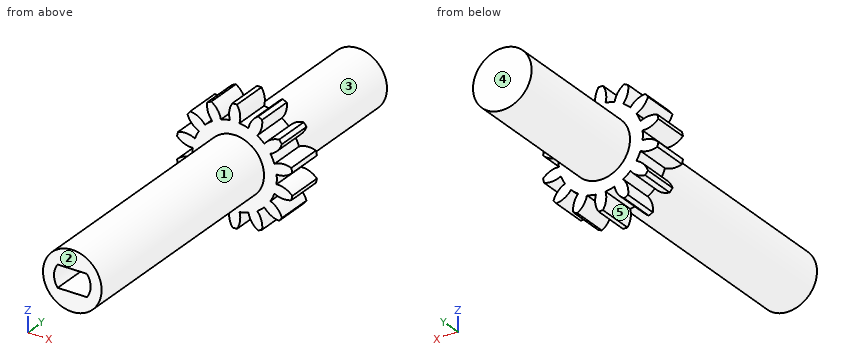
```python
from build123d import *

# Parameters (mm, degrees)
SKETCH1_R                = 0.4
BOSS_EXTRUDE1_DEPTH      = 5
BOSS_EXTRUDE2_DEPTH      = 33
BOSS_EXTRUDE2_DEPTH_BACK = 5
SKETCH2_R                = 4
BOSS_EXTRUDE3_START      = 20
SKETCH3_R                = 4
BOSS_EXTRUDE3_DEPTH      = 20
CUT_EXTRUDE1_DEPTH       = 33


with BuildPart() as part:
    # Sketch1 → Boss-Extrude1 (new body)
    with BuildSketch(Plane(origin=(0, 0, 0), x_dir=(1, 0, 0), z_dir=(0, 1, 0))):
        with BuildLine():
            ThreePointArc((3.744900382, -7.069350828), (3.64692573, -5.891768521), (3.071904032, -4.859465672))
            ThreePointArc((3.071904032, -4.859465672), (3.584442871, -4.494749193), (4.054065768, -4.076217824))
            ThreePointArc((4.054065768, -4.076217824), (4.932532263, -4.866531521), (6.058788713, -5.224086459))
            ThreePointArc((6.058788713, -5.224086459), (6.25465186, -4.987918415), (6.441315028, -4.744413632))
            ThreePointArc((6.441315028, -4.744413632), (5.842109102, -3.725958242), (4.876133034, -3.045378078))
            ThreePointArc((4.876133034, -3.045378078), (5.179670022, -2.494397616), (5.421191676, -1.913552144))
            ThreePointArc((5.421191676, -1.913552144), (6.555566902, -2.244447854), (7.725426174, -2.077929362))
            ThreePointArc((7.725426174, -2.077929362), (7.799423297, -1.780167472), (7.861948235, -1.47978713))
            ThreePointArc((7.861948235, -1.47978713), (6.880191117, -0.822176238), (5.714584087, -0.628116006))
            ThreePointArc((5.714584087, -0.628116006), (5.749, 0), (5.714584087, 0.628116006))
            ThreePointArc((5.714584087, 0.628116006), (6.880191117, 0.822176238), (7.861948235, 1.47978713))
            ThreePointArc((7.861948235, 1.47978713), (7.799423297, 1.780167472), (7.725426174, 2.077929362))
            ThreePointArc((7.725426174, 2.077929362), (6.555566902, 2.244447854), (5.421191676, 1.913552144))
            ThreePointArc((5.421191676, 1.913552144), (5.179670022, 2.494397616), (4.876133034, 3.045378078))
            ThreePointArc((4.876133034, 3.045378078), (5.842109102, 3.725958242), (6.441315028, 4.744413632))
            ThreePointArc((6.441315028, 4.744413632), (6.25465186, 4.987918415), (6.058788713, 5.224086459))
            ThreePointArc((6.058788713, 5.224086459), (4.932532263, 4.866531521), (4.054065768, 4.076217824))
            ThreePointArc((4.054065768, 4.076217824), (3.584442871, 4.494749193), (3.071904032, 4.859465672))
            ThreePointArc((3.071904032, 4.859465672), (3.64692573, 5.891768521), (3.744900382, 7.069350828))
            ThreePointArc((3.744900382, 7.069350828), (3.471069913, 7.207750943), (3.192133841, 7.335549164))
            ThreePointArc((3.192133841, 7.335549164), (2.332549116, 6.524738937), (1.883982415, 5.431538572))
            ThreePointArc((1.883982415, 5.431538572), (1.279272849, 5.604860567), (0.659246762, 5.711076493))
            ThreePointArc((0.659246762, 5.711076493), (0.72942399, 6.890641786), (0.306762287, 7.994116393))
            ThreePointArc((0.306762287, 7.994116393), (0, 8), (-0.306762287, 7.994116393))
            ThreePointArc((-0.306762287, 7.994116393), (-0.72942399, 6.890641786), (-0.659246762, 5.711076493))
            ThreePointArc((-0.659246762, 5.711076493), (-1.279272849, 5.604860567), (-1.883982415, 5.431538572))
            ThreePointArc((-1.883982415, 5.431538572), (-2.332549116, 6.524738937), (-3.192133841, 7.335549164))
            ThreePointArc((-3.192133841, 7.335549164), (-3.471069913, 7.207750943), (-3.744900382, 7.069350828))
            ThreePointArc((-3.744900382, 7.069350828), (-3.64692573, 5.891768521), (-3.071904032, 4.859465672))
            ThreePointArc((-3.071904032, 4.859465672), (-3.584442871, 4.494749193), (-4.054065768, 4.076217824))
            ThreePointArc((-4.054065768, 4.076217824), (-4.932532263, 4.866531521), (-6.058788713, 5.224086459))
            ThreePointArc((-6.058788713, 5.224086459), (-6.25465186, 4.987918415), (-6.441315028, 4.744413632))
            ThreePointArc((-6.441315028, 4.744413632), (-5.842109102, 3.725958242), (-4.876133034, 3.045378078))
            ThreePointArc((-4.876133034, 3.045378078), (-5.179670022, 2.494397616), (-5.421191676, 1.913552144))
            ThreePointArc((-5.421191676, 1.913552144), (-6.555566902, 2.244447854), (-7.725426174, 2.077929362))
            ThreePointArc((-7.725426174, 2.077929362), (-7.799423297, 1.780167472), (-7.861948235, 1.47978713))
            ThreePointArc((-7.861948235, 1.47978713), (-6.880191117, 0.822176238), (-5.714584087, 0.628116006))
            ThreePointArc((-5.714584087, 0.628116006), (-5.749, 0), (-5.714584087, -0.628116006))
            ThreePointArc((-5.714584087, -0.628116006), (-6.880191117, -0.822176238), (-7.861948235, -1.47978713))
            ThreePointArc((-7.861948235, -1.47978713), (-7.799423297, -1.780167472), (-7.725426174, -2.077929362))
            ThreePointArc((-7.725426174, -2.077929362), (-6.555566902, -2.244447854), (-5.421191676, -1.913552144))
            ThreePointArc((-5.421191676, -1.913552144), (-5.179670022, -2.494397616), (-4.876133034, -3.045378078))
            ThreePointArc((-4.876133034, -3.045378078), (-5.842109102, -3.725958242), (-6.441315028, -4.744413632))
            ThreePointArc((-6.441315028, -4.744413632), (-6.25465186, -4.987918415), (-6.058788713, -5.224086459))
            ThreePointArc((-6.058788713, -5.224086459), (-4.932532263, -4.866531521), (-4.054065768, -4.076217824))
            ThreePointArc((-4.054065768, -4.076217824), (-3.584442871, -4.494749193), (-3.071904032, -4.859465672))
            ThreePointArc((-3.071904032, -4.859465672), (-3.64692573, -5.891768521), (-3.744900382, -7.069350828))
            ThreePointArc((-3.744900382, -7.069350828), (-3.471069913, -7.207750943), (-3.192133841, -7.335549164))
            ThreePointArc((-3.192133841, -7.335549164), (-2.332549116, -6.524738937), (-1.883982415, -5.431538572))
            ThreePointArc((-1.883982415, -5.431538572), (-1.279272849, -5.604860567), (-0.659246762, -5.711076493))
            ThreePointArc((-0.659246762, -5.711076493), (-0.72942399, -6.890641786), (-0.306762287, -7.994116393))
            ThreePointArc((-0.306762287, -7.994116393), (0, -8), (0.306762287, -7.994116393))
            ThreePointArc((0.306762287, -7.994116393), (0.72942399, -6.890641786), (0.659246762, -5.711076493))
            ThreePointArc((0.659246762, -5.711076493), (1.279272849, -5.604860567), (1.883982415, -5.431538572))
            ThreePointArc((1.883982415, -5.431538572), (2.332549116, -6.524738937), (3.192133841, -7.335549164))
            ThreePointArc((3.192133841, -7.335549164), (3.471069913, -7.207750943), (3.744900382, -7.069350828))
        make_face()
        with Locations(Location((0, 0, 0), (0, 0, 90))):
            Circle(SKETCH1_R, mode=Mode.SUBTRACT)
    extrude(amount=-BOSS_EXTRUDE1_DEPTH)

    # Sketch2 → Boss-Extrude2 (add, two sides: drawn at the far end of the back side and taken through both)
    with BuildSketch(Plane.XZ.offset(5).offset(-BOSS_EXTRUDE2_DEPTH_BACK)):
        with Locations(Location((0, 0, 0), (0, 0, 270))):
            Circle(SKETCH2_R)
    extrude(amount=BOSS_EXTRUDE2_DEPTH + BOSS_EXTRUDE2_DEPTH_BACK)

    # Sketch3 → Boss-Extrude3 (add)
    with BuildSketch(Plane(origin=(0, 0, 0), x_dir=(1, 0, 0), z_dir=(0, 1, 0)).offset(BOSS_EXTRUDE3_START)):
        with Locations(Location((0, 0, 0), (0, 0, 90))):
            Circle(SKETCH3_R)
    extrude(amount=-BOSS_EXTRUDE3_DEPTH)

    # Sketch4 → Cut-Extrude1 (cut)
    with BuildSketch(Plane.XZ.offset(38)):
        with BuildLine():
            Line((-2, -1.5), (2, -1.5))
            ThreePointArc((2, -1.5), (2.5, 0), (2, 1.5))
            Line((2, 1.5), (-2, 1.5))
            ThreePointArc((-2, 1.5), (-2.5, 0), (-2, -1.5))
        make_face()
    extrude(amount=-CUT_EXTRUDE1_DEPTH, mode=Mode.SUBTRACT)


solid = part.part
```
The model under review builds one solid part; all positions refer to its coordinate system, in mm. Face numbers are marked on the shaded views. A direction names the side the tool comes from. Give positions to 0.01 mm unless a question says otherwise; leave off trailing zeros. Loops run counter-clockwise (first coordinate to the right, second up) from the corner with the lowest first, then second, coordinate; pieces in that order, holes last. Notation, with made-up numbers: (10.5, 32.25) - (24.5, 32.25) arc R18 cw to (24.5, 47.25) - close; hole circle Ø5 at (84.5, 21). An arc over 180 degrees is marked (long way). Answer as a JSON object with one key per item and string values.
Q1. Add section C-C on y = 14.5. State the section outline as (x, z) points.
Worked out:
{"outline": "circle Ø8 at (0, 0)"}
Q2. To check wall thickness, follow line 1 along X through (y, z) = (-2, 7); line 2 along X through (y, z) = (-3, 5.75); line 3 along Y through (x, z) = (-2, -4.25). State the ranges of each line that lie inside material, in increasing order.
Worked out:
{"line 1": "x = -3.75 to -2.74, -0.71 to 0.71, 2.74 to 3.75", "line 2": "x = -3.6 to -1.96, -0.67 to 0.67, 1.96 to 3.6", "line 3": "y = -5 to 0"}
Q3. Insertion check: pin 1 (8 mm diameter, centred on x = 5.5, y = -6.5, fed in from +Z); pin 2 (2 mm diameter, centred on y = -9, z = -1.5, fed in from -X); pin 3 (1 mm diameter, centred on y = -4.5, z = -5.5, fed in from +X) (3 decimals). Each pin has a flat end and moves straight along its axis. Give the tip position at first contact, or say it passes through.
Worked out:
{"pin 1": "stops at z = 7.34", "pin 2": "stops at x = -3.97", "pin 3": "stops at x = 6.245"}
Q4. Mouldability with a two-part tool opening along X and no side actions: class the marked faces 3, 4 and 5 as +X half, -X half, draft (parallel to the pull), parting line (faces both ways), or undercut.
Worked out:
{"face 3": "parting line", "face 4": "draft", "face 5": "undercut"}
Q5. Add section B-B on z = 0. State the section outline as (x, y) points, plus the area to 3 significant figures.
Worked out:
{"outline": "(-5.75, -5) - (-4, -5) - (-4, -38) - (-2.5, -38) - (-2.5, -5) - (2.5, -5) - (2.5, -38) - (4, -38) - (4, -5) - (5.75, -5) - (5.75, 0) - (4, 0) - (4, 20) - (-4, 20) - (-4, 0) - (-5.75, 0) - close", "area": "316 mm^2"}
Q6. For the marked faces 1 and 2, list the 3-axis set-ups (+Z, -Z, +X, -X, +Y, -Y) from which the entire face can be reached by the end or side of a thin tool; tool diameter is ignored.
Worked out:
{"face 1": "-Y", "face 2": "+Z, -Z, +X, -X, -Y"}
Q7. Add section A-A on z = 6.25. State the section outline as (x, y) points, plus the area to 3 significant figures.
Worked out:
{"outline": "(-3.73, -5) - (-2.17, -5) - (-2.17, 0) - (-3.73, 0) - close; (-0.75, -5) - (0.75, -5) - (0.75, 0) - (-0.75, 0) - close; (2.17, -5) - (3.73, -5) - (3.73, 0) - (2.17, 0) - close", "area": "23.2 mm^2"}
